Part model, mm, in its own coordinate system. Face numbers are marked on the shaded views. A direction names the side the tool comes from. Round coordinates to 2 decimals unless told otherwise and drop trailing zeros. Loops run counter-clockwise (first coordinate to the right, second up) from the corner with the lowest first, then second, coordinate; pieces in that order, holes last. Notation, with made-up numbers: (6.5, 21) -> (18.5, 21) arc R26 cw to (18.5, 47) -> close; hole circle Ø10 at (-15.75, -26). An arc over 180 degrees is marked (long way). Answer as CSV lines item,"result".
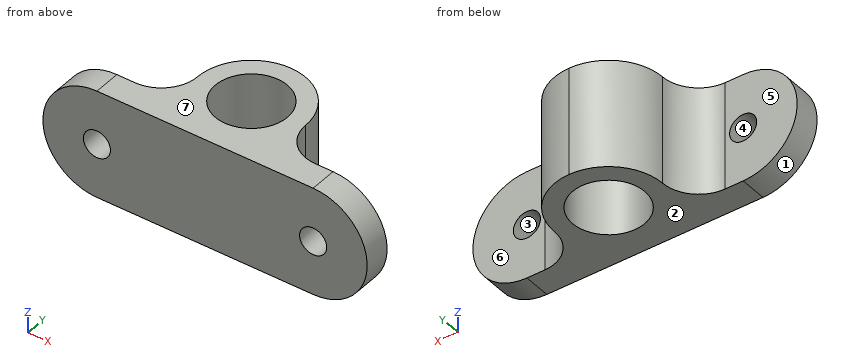
from build123d import *

# Parameters (mm, degrees)
BOSS_EXTRUDE1_DEPTH = 4.7752
SKETCH3_R           = 2.3876
CUT_EXTRUDE1_DEPTH  = 52.515489516
SKETCH4_W           = 19.05
SKETCH4_H           = 19.05
BOSS_EXTRUDE2_DEPTH = 15.8496
SKETCH5_R           = 6.35
CUT_EXTRUDE3_DEPTH  = 56.284948223
FILLET1_R           = 6.35
FILLET2_R           = 6.35


with BuildPart() as part:
    # Sketch1 → Boss-Extrude1 (new body)
    with BuildSketch(Plane(origin=(0, 0, 0), x_dir=(1, 0, 0), z_dir=(0, 1, 0))):
        with BuildLine():
            Line((0, 19.05), (38.1, 19.05))
            ThreePointArc((38.1, 19.05), (47.625, 9.525), (38.1, 0))
            Line((38.1, 0), (0, 0))
            ThreePointArc((0, 0), (-9.525, 9.525), (0, 19.05))
        make_face()
    extrude(amount=BOSS_EXTRUDE1_DEPTH)

    # Sketch3 → Cut-Extrude1 (cut, through all)
    with BuildSketch(Plane(origin=(0, 4.7752, 0), x_dir=(1, 0, 0), z_dir=(0, 1, 0))):
        with Locations(Location((38.1, 9.525, 0), (0, 0, 270))):
            Circle(SKETCH3_R)
        with Locations(Location((0, 9.525, 0), (0, 0, 270))):
            Circle(SKETCH3_R)
    extrude(amount=-CUT_EXTRUDE1_DEPTH, mode=Mode.SUBTRACT)

    # Sketch4 → Boss-Extrude2 (add)
    with BuildSketch(Plane(origin=(0, 4.7752, 0), x_dir=(1, 0, 0), z_dir=(0, 1, 0))):
        with Locations((19.05, 9.525)):
            Rectangle(SKETCH4_W, SKETCH4_H)
    extrude(amount=BOSS_EXTRUDE2_DEPTH)

    # Sketch5 → Cut-Extrude3 (cut, through all)
    with BuildSketch(Plane.XY):
        with BuildLine():
            ThreePointArc((19.05, 20.6248), (25.785192091, 17.834992091), (28.575, 11.0998))
            Line((28.575, 11.0998), (28.575, 20.6248))
            Line((28.575, 20.6248), (19.05, 20.6248))
        make_face()
        with BuildLine():
            ThreePointArc((9.525, 11.0998), (12.314807909, 17.834992091), (19.05, 20.6248))
            Line((19.05, 20.6248), (9.525, 20.6248))
            Line((9.525, 20.6248), (9.525, 11.0998))
        make_face()
        with Locations((19.05, 11.0998)):
            Circle(SKETCH5_R)
    extrude(amount=-CUT_EXTRUDE3_DEPTH, mode=Mode.SUBTRACT)

    # Fillet1
    fillet1_edges = [part.edges().sort_by_distance(p)[0] for p in [
        (28.575, 4.7752, -9.525),
    ]]
    fillet(fillet1_edges, radius=FILLET1_R)

    # Fillet2
    fillet2_edges = [part.edges().sort_by_distance(p)[0] for p in [
        (9.525, 4.7752, -9.525),
    ]]
    fillet(fillet2_edges, radius=FILLET2_R)


solid = part.part
Q1. Saw through at C-C, the plane z = -11. Give the number of separate pieces and of enclosed holes in the cut face, then the cut area to 3 significant figures.
Geometry results:
separate pieces,"3"
enclosed holes,"1"
area,"390 mm2"
Q2. Saw through at B-B, the plane x = 17. Write the cut outline in (y, z), then the cut area to 3 significant figures.
Geometry results:
outline,"(0, -19.05) -> (5.09, -19.05) -> (5.09, 0) -> (0, 0) -> close; (17.11, -19.05) -> (20.4, -19.05) -> (20.4, 0) -> (17.11, 0) -> close"
area,"160 mm2"
Q3. Saw through at A-A, the plane y = 1.5. Write the cut outline in (x, z) (3 decimals), then the cut area to 3 significant figures.
Geometry results:
outline,"(0, -19.05) -> (38.1, -19.05) arc R9.525 ccw to (38.1, 0) -> (0, 0) arc R9.525 ccw to start; hole circle Ø4.775 at (0, -9.525); hole circle Ø4.775 at (38.1, -9.525)"
area,"975 mm2"
Q4. Which spindle directions (+Z, -Z, +X, -X, +Y, -Y) get a long thin tool onto all of the face, cutting with end or side? Do the marked faces 5, 6 and 7. Say none if no direction does.
Geometry results:
face 5,"+Z, -Z, -X, +Y"
face 6,"+Z, -Z, +X, +Y"
face 7,"+Z, +X, -X, +Y, -Y"
Q5. Two-plate mould, pull along X, no slides. Class the marked faces 1, 2, 3 and 4: pulls with the +X half, pulls with the -X half, needs draft (parallel to the pull), parting line crosses it, or undercut.
Geometry results:
face 1,"pulls with the -X half"
face 2,"needs draft"
face 3,"undercut"
face 4,"undercut"
Q6. Drill centre lines: line 1 along X through (y, z) = (11.5, -8.25); line 2 along Y through (x, z) = (19.05, -8); line 3 along X through (y, z) = (3.5, -7.75). Where is each one in solid material? Low to high.
Geometry results:
line 1,"9.53 to 12.71, 25.39 to 28.57"
line 2,"0 to 4.75, 17.45 to 20.62"
line 3,"-9.36 to -1.6, 1.6 to 36.5, 39.7 to 47.46"
Q7. Saw through at D-D, the plane y = 12. Write the cut outline in (x, z).
Geometry results:
outline,"(9.57, -19.05) -> (12.76, -19.05) -> (12.76, 0) -> (9.57, 0) -> close; (25.34, -19.05) -> (28.53, -19.05) -> (28.53, 0) -> (25.34, 0) -> close"
Q8. Drop flat-ended pins along their axis: P1, Ø4, axis at x = 38.1, z = -9.525, coming from the -Y side; P2, Ø1.5, axis at y = 11.5, z = -5.5, coming from the -X side; P3, Ø6.5, axis at x = 41.5, z = -9, coming from the +Y side; P4, Ø1, axis at y = 2.5, z = -15, coming from the -X side. Give the stop position or say it passes through.
Geometry results:
P1,"through"
P2,"x = 9.51"
P3,"y = 4.78"
P4,"x = -8.12"
